Design review of the part built by this model. Coordinates are the model's own, in mm. A direction names the side the tool comes from. Give positions to 0.01 mm unless a question says otherwise; leave off trailing zeros. Write each loop counter-clockwise with the first axis right and the second up, starting at its lowest first coordinate (ties: lowest second). Pieces come first, ordered by that corner, then holes.
```python
from build123d import *

# Parameters (mm, degrees)
SKETCH_1_W          = 50
SKETCH_1_H          = 20
EXTRUDE_1_DEPTH     = 3
SKETCH_2_R          = 5
SKETCH_2_W          = 30
SKETCH_2_H          = 7
CUT_EXTRUDE_1_DEPTH = 3


with BuildPart() as part:
    # 스케치1 → 보스-돌출1 (new body)
    with BuildSketch(Plane.XY):
        Rectangle(SKETCH_1_W, SKETCH_1_H)
    extrude(amount=EXTRUDE_1_DEPTH)

    # 스케치2 → 컷-돌출1 (cut)
    with BuildSketch(Plane.XY.offset(3)):
        with Locations((-15, 0)):
            Circle(SKETCH_2_R)
        with Locations((15, 0)):
            Circle(SKETCH_2_R)
        Rectangle(SKETCH_2_W, SKETCH_2_H)
    extrude(amount=-CUT_EXTRUDE_1_DEPTH, mode=Mode.SUBTRACT)


solid = part.part
```
(1) Clearance check with a flat-ended pin moving along its axis: P1, Ø9, axis at x = -15, y = 0, coming from the -Z side. State where the tip first meets the part, or that it passes through.
Resolved:
P1: passes through
(2) Mouldability with a two-part tool opening along X and no side actions: class faces 1 (the face through (25, 0, 1)), 2 (the face through (0, 5, 3)), 3 (the face through (20, 0, 2)) as pulls with the +X half, pulls with the -X half, needs draft (parallel to the pull), parting line crosses it, or undercut.
Resolved:
face 1: pulls with the +X half
face 2: needs draft
face 3: undercut
(3) Consider section A-A, the plane x = 0.5. Give the boundary of the cut face in (y, z).
Resolved:
outline: (-10, 0) - (-3.5, 0) - (-3.5, 3) - (-10, 3) - close; (3.5, 0) - (10, 0) - (10, 3) - (3.5, 3) - close
(4) Consider section C-C, the plane z = 0.8. Give the boundary of the cut face in (x, y).
Resolved:
outline: (-25, -10) - (25, -10) - (25, 10) - (-25, 10) - close; hole (-11.43, -3.5) - (11.43, -3.5) arc R5 ccw (long way) to (11.43, 3.5) - (-11.43, 3.5) arc R5 ccw (long way) to start
(5) To check wall thickness, follow L1, parallel to Y at x = 11, z = 1.6; L2, parallel to Y at x = -15, z = 1.35; L3, parallel to X at y = 1, z = 2.8. State the ranges of each line that lie inside material, in increasing order.
Resolved:
L1: y = -10 to -3.5, 3.5 to 10
L2: y = -10 to -5, 5 to 10
L3: x = -25 to -19.9, 19.9 to 25
(6) Tool access review of faces 4 (the face through (0, 10, 1)), 5 (the face through (0, -3.5, 2)): name each direction out of +Z, -Z, +X, -X, +Y, -Y from which nothing blocks a thin tool from reaching the whole face with its end or side.
Resolved:
face 4: +Z, -Z, +X, -X, +Y
face 5: +Z, -Z
(7) Consider section B-B, the plane y = -3. Give the boundary of the cut face in (x, z), then the cut area to 3 significant figures.
Resolved:
outline: (-25, 0) - (-19, 0) - (-19, 3) - (-25, 3) - close; (19, 0) - (25, 0) - (25, 3) - (19, 3) - close
area: 36.0 mm2
